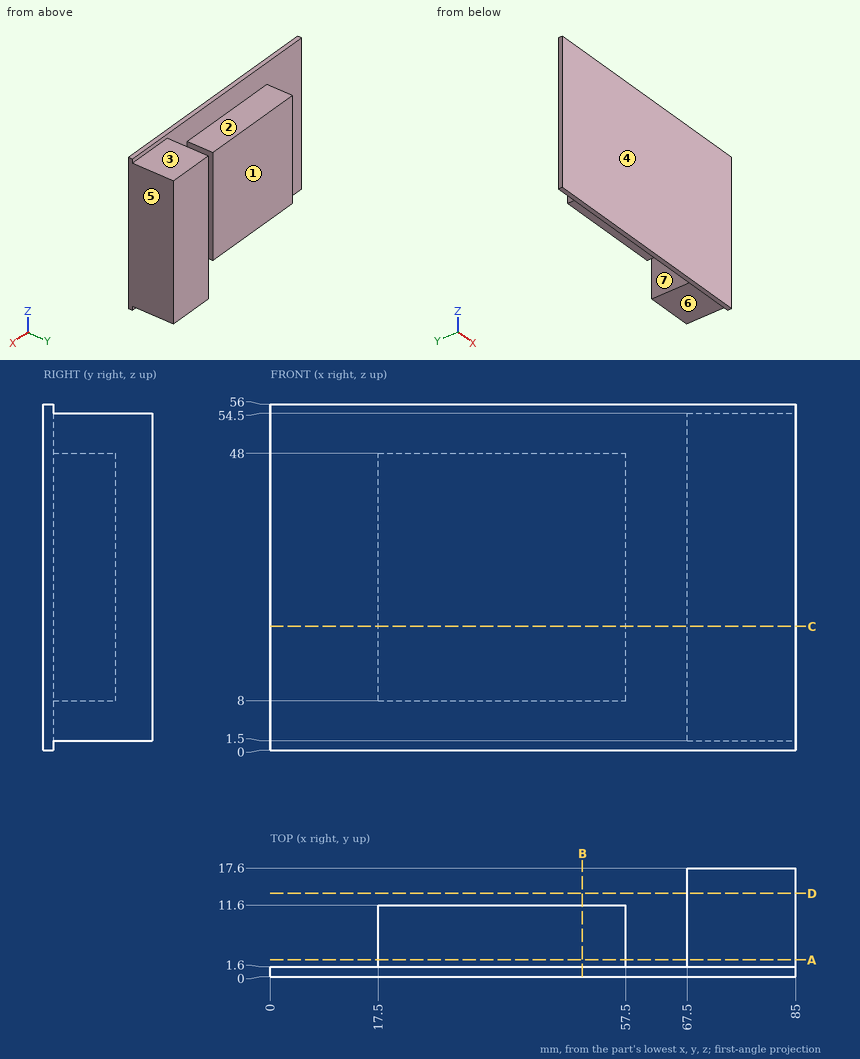
Study the drawing (mm; zero at the part's minimum x, y, z) and answer. A direction names the side the tool comes from. Coordinates: 2 decimals unless noted, no trailing zeros. Write each loop counter-clockwise with the first axis right and the second up, starting at its lowest first coordinate (ties: lowest second). Pieces come first, ordered by that corner, then holes. Notation, with made-up numbers: (9, -18) - (24, -18) arc R11 cw to (24, -12) - close; hole circle Ø10 at (28.25, 53). An arc over 180 degrees is marked (long way). One line per question, with ' | ' between items.
1) Find section D-D, the plane y = 13.5. Determine the outline of the cut face in (x, z).
Checks:
outline: (67.5, 1.5) - (85, 1.5) - (85, 54.5) - (67.5, 54.5) - close
2) Consider probe 1 along X at (y, z) = (3.5, 30.5); probe 2 along Z at (x, y) = (37.5, 8.75); probe 3 along Y at (x, z) = (16, 32.5). Determine where each line is inside the solid, lowest interval first. Write a range as [from, to].
Checks:
probe 1: [17.5, 57.5], [67.5, 85] | probe 2: [8, 48] | probe 3: [0, 1.6]
3) Find section B-B, the plane x = 50.5. Determine the outline of the cut face in (y, z).
Checks:
outline: (0, 0) - (1.6, 0) - (1.6, 8) - (11.6, 8) - (11.6, 48) - (1.6, 48) - (1.6, 56) - (0, 56) - close
4) Flat-ended cylindrical pins translate along their axes: P1, Ø3, axis at x = 38.5, y = 8, coming from the -Z side; P2, Ø8, axis at y = 12, z = 39, coming from the -X side; P3, Ø20, axis at x = 41.5, z = 33.5, coming from the +Y side. Find the tip coordinate at first contact, or state that the pin passes through.
Checks:
P1: z = 8 | P2: x = 17.5 | P3: y = 11.6
5) Find section A-A, the plane y = 2.75. Determine the outline of the cut face in (x, z).
Checks:
outline: (17.5, 8) - (57.5, 8) - (57.5, 48) - (17.5, 48) - close; (67.5, 1.5) - (85, 1.5) - (85, 54.5) - (67.5, 54.5) - close
6) Find section C-C, the plane z = 20. Determine the outline of the cut face in (x, y).
Checks:
outline: (0, 0) - (85, 0) - (85, 17.6) - (67.5, 17.6) - (67.5, 1.6) - (57.5, 1.6) - (57.5, 11.6) - (17.5, 11.6) - (17.5, 1.6) - (0, 1.6) - close
7) The mould has two halves that part along X. Classify the marked faces 5, 6 and 7: +X half, -X half, draft (parallel to the pull), parting line (faces both ways), or undercut.
Checks:
face 5: +X half | face 6: draft | face 7: undercut
8) For the marked faces 1, 2, 3 and 4, determine the directions among +Z, -Z, +X, -X, +Y, -Y from which every point of the face is accessible in a straight line to the end or side of a thin tool.
Checks:
face 1: +Z, -Z, -X, +Y | face 2: +Z, -X, +Y | face 3: +Z, +X, -X, +Y | face 4: +Z, -Z, +X, -X, -Y
